Autodesk Inventor part; units mm, degrees
ref_plane "Plano de trabajo1" through (-18, 0, -54) normal (1, 0, 0) x (0, 0, -1)
ref_plane "YZ Plane" through (0, 0, 0) normal (1, 0, 0) x (0, 1, 0)
ref_plane "XZ Plane" through (0, 0, 0) normal (0, 1, 0) x (-1, 0, 0)
sketch "Boceto1" plane through (0, 0, 0) normal (0, 1, 0) x (-1, 0, 0)
  line L0 (-15, 60) -> (15, 60)
  line L1 (21, 54) -> (21, -54)
  line L2 (15, -60) -> (-15, -60)
  line L3 (-21, -54) -> (-21, 54)
  line L4 (-21, 60) -> (21, -60) construction
  line L5 (21, 60) -> (-21, -60) construction
  arc A0 (21, 54) -> (15, 60) centre (15, 54) ccw
  arc A1 (-15, 60) -> (-21, 54) centre (-15, 54) ccw
  arc A2 (-21, -54) -> (-15, -60) centre (-15, -54) ccw
  arc A3 (15, -60) -> (21, -54) centre (15, -54) ccw
  circle A4 centre (0, 46) radius 7.5
  circle A5 centre (0, -46) radius 7.5
  point P0 (0, 0)
  dimension "d0" = 42
  dimension "d1" = 120
  dimension "d2" = 6
  dimension "d3" = 15
  dimension "d13" = 46
  dimension "d14" = 46
extrude "Extrusión1" add sketch "Boceto1" along normal blind 10
sketch "Boceto2" plane through (-21, 0, -54) normal (-1, 0, 0) x (0, 0, 1)
  line L0 (0, 10) -> (108, 10) construction
  line L1 (24, 86.9722) -> (24, 26)
  line L2 (84, 86.9722) -> (84, 26)
  line L3 (0, 0) -> (108, 0)
  arc A0 (84, 26) -> (100, 10) centre (100, 26) ccw
  arc A1 (8, 10) -> (24, 26) centre (8, 26) ccw
  line L4 (92.5, 10) -> (107.5, 10) construction
  line L5 (0.5, 10) -> (15.5, 10) construction
  circle A2 centre (54, 105) radius 35
  line L6 (8, 10) -> (100, 10)
  point P0 (54, 0)
  point P1 (24, 10)
  point P2 (84, 10)
  point P3 (54, 0)
  point P4 (54, 0)
  point P5 (54, 10)
  dimension "d10" = 16
  dimension "d16" = 35
  dimension "d17" = 95
extrude "Extrusión2" add sketch "Boceto2" against normal blind 6 contours A2 L2 A0 L6 A1 L1
ref_plane "Plano de trabajo1" through (-18, 0, -54) normal (1, 0, 0) x (0, 0, -1)
sketch "Boceto3" plane through (-18, 0, -54) normal (1, 0, 0) x (0, 0, -1)
  arc A0 (-84, 86.9722) -> (-24, 86.9722) centre (-54, 105) ccw
  circle A1 centre (-54, 105) radius 35
  circle A2 centre (-54, 105) radius 30
  line L0 (-57, 10) -> (-51, 10)
  line L1 (-51, 10) -> (-51, 70.1288)
  line L2 (-51, 70.1288) -> (-57, 70.1288)
  line L3 (-57, 70.1288) -> (-57, 10)
  line L4 (-57, 10) -> (-51, 70.1288) construction
  line L5 (-51, 10) -> (-57, 70.1288) construction
  line L6 (-8, 10) -> (-100, 10)
  line L7 (-55.5, 105) -> (-52.5, 105)
  line L8 (-52.5, 105) -> (-52.5, 175)
  line L9 (-52.5, 175) -> (-55.5, 175)
  line L10 (-55.5, 175) -> (-55.5, 105)
  line L11 (-55.5, 105) -> (-52.5, 175) construction
  line L12 (-52.5, 105) -> (-55.5, 175) construction
  point P0 (-54, 0)
  point P1 (-54, 40.0644)
  point P2 (-54, 140)
  point P3 (-55.5, 134.9625)
  point P4 (-55.5, 139.9678)
  point P5 (-52.5, 139.9678)
  point P6 (-52.5, 134.9625)
  dimension "d23" = 39
  dimension "d20" = 30
  dimension "d21" = 6
  dimension "d22" = 3
extrude "Extrusión3" add sketch "Boceto3" along normal up to surface (39 mm away) contours A1 L10 A2 L8 A0 L2 | L2 A0 | A0 L1 L0 L3
sketch "Boceto4" plane through (-18, 0, -54) normal (-1, 0, 0) x (0, 0, 1)
  arc A0 (24, 86.9722) -> (84, 86.9722) centre (54, 105) ccw
  arc A1 (84, 86.9722) -> (55.5, 139.9678) centre (54, 105) ccw
  line L0 (55.5, 134.9625) -> (55.5, 139.9678)
  arc A2 (52.5, 134.9625) -> (55.5, 134.9625) centre (54, 105) ccw
  line L1 (52.5, 139.9678) -> (52.5, 134.9625)
  arc A3 (52.5, 139.9678) -> (24, 86.9722) centre (54, 105) ccw
  point P0 (54, 0)
extrude "Extrusión4" add sketch "Boceto4" along normal blind 9
sketch "Sketch6" plane through (-21, 0, -54) normal (-1, 0, 0) x (0, 0, 1)
  arc A0 (52.5, 139.9678) -> (55.5, 139.9678) centre (54, 105) ccw
  line L0 (52.5, 139.9678) -> (52.5, 161)
  line L1 (52.5, 161) -> (21.5, 161)
  line L2 (21.5, 161) -> (21.5, 117.9904)
  line L3 (21.5, 147) -> (52.5, 147) construction
  point P0 (54, 0)
  dimension "d30" = 31
  dimension "d31" = 42
  dimension "d32" = 14
extrude "Extrusion5" add sketch "Sketch6" against normal blind 28
fillet "Fillet1" radius 14 2 edges at (7, 161, -17) (-21, 161, -17)
sketch "Sketch7" plane through (7, 117.9904, -32.5) normal (0, 0, -1) x (-1, 0, 0)
  arc A0 (28, 29.0096) -> (0, 29.0096) centre (14, 29.0096) ccw
  point P0 (7, -117.9904)
hole "Hole1" at (-7, 147, -32.5) direction (0, 0, 1) diameter 12 depth 31
mirror "Mirror1" about plane through (0, 0, 0) normal (0, 0, 1) of "Extrusion5", "Fillet1", "Hole1"
sketch "Sketch8" plane through (0, 0, 0) normal (0, 0, 1) x (1, 0, 0)
  line L0 (-27, 70) -> (-21, 70)
  line L1 (-21, 0) -> (-21, 10)
  line L2 (-21, 10) -> (-21, 26)
  line L3 (-21, 26) -> (-21, 86.9722)
  line L4 (-21, 86.9722) -> (-21, 86.9722)
  line L5 (-21, 86.9722) -> (-21, 26)
  line L6 (-21, 26) -> (-21, 10)
  line L7 (-21, 0) -> (-21, 10)
  line L8 (-27, 70) -> (-21, 20)
  line L9 (-27, 139.9678) -> (-27, 70)
  line L10 (-27, 70) -> (-27, 73)
  line L11 (-27, 73) -> (-21, 73)
  point P0 (0, 0)
  dimension "d43" = 20
  dimension "d44" = 3
extrude "Extrusion6" add sketch "Sketch8" along normal mid plane 6
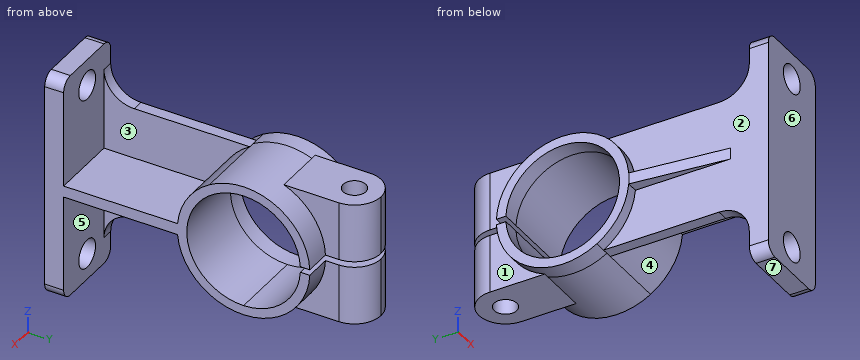
Input: part model. Units: mm. Frame: model coordinates. Face numbers are marked on the shaded views. A direction names the side the tool comes from. Coordinates: 2 decimals unless noted, no trailing zeros. Loops run counter-clockwise (first coordinate to the right, second up) from the corner with the lowest first, then second, coordinate; pieces in that order, holes last. Notation, with made-up numbers: (80.25, -36.75) -> (137.25, -36.75) arc R14 ccw to (137.25, -25.75) -> close; hole circle Ø10 at (75, 71.5). An arc over 180 degrees is marked (long way). Use a Markdown table: item, result.
1) Pull-direction query (Y, two-part tool) for the marked faces 5, 6 and 7; classes: released by +Y, released by -Y, zero draft, split by the parting line, or undercut.
Results found:
| item | result |
|---|---|
| face 5 | undercut |
| face 6 | released by -Y |
| face 7 | zero draft |
2) Cut plane D-D (y = 100.5). Return the cut outline in (x, z).
Results found:
| item | result |
|---|---|
| outline | (-27, -34.71) -> (21, -34.71) -> (21, -29.66) -> (-27, -29.66) -> close; (-27, 29.66) -> (21, 29.66) -> (21, 34.71) -> (-27, 34.71) -> close |
3) Access query for the marked faces 1, 2, 3 and 4. Directions: +Z, -Z, +X, -X, +Y, -Y. A direction counts if a zero-diameter tool reaches every point of the face in a straight line with its end or side. Return the directions, or none.
Results found:
| item | result |
|---|---|
| face 1 | -Z, -X, +Y |
| face 2 | -X, -Y |
| face 3 | +Z, +X |
| face 4 | -Z, +X |
4) Cut plane B-B (x = 2). Return the cut outline in (y, z).
Results found:
| item | result |
|---|---|
| outline | (0, -60) -> (10, -60) -> (10, -53.23) -> (0, -53.23) -> close; (0, -38.77) -> (10, -38.77) -> (10, -3) -> (70.13, -3) arc R35 ccw to (117.99, -32.5) -> (157.72, -32.5) -> (157.72, -1.5) -> (134.96, -1.5) arc R30 cw (long way) to (134.96, 1.5) -> (157.72, 1.5) -> (157.72, 32.5) -> (117.99, 32.5) arc R35 ccw to (86.97, 30) arc R35 ccw to (70.13, 3) -> (10, 3) -> (10, 38.77) -> (0, 38.77) -> close; (0, 53.23) -> (10, 53.23) -> (10, 60) -> (0, 60) -> close |
5) Contact query for flat-ended pins moving along their axis: pin 1 (1.5 mm diameter, centred on x = 10.5, z = 42, fed in from +Y); pin 2 (21 mm diameter, centred on x = -7.5, z = 38, fed in from +Y); pin 3 (19 mm diameter, centred on x = -7, y = 147, fed in from -Z); pin 4 (3 mm diameter, centred on x = -24.5, y = 56.5, fed in from +Z). Output: stop coordinate, or through.
Results found:
| item | result |
|---|---|
| pin 1 | stops at y = 10 |
| pin 2 | stops at y = 161 |
| pin 3 | stops at z = -32.5 |
| pin 4 | stops at z = 3 |
6) Cut plane C-C (y = 129.5). Return the cut outline in (x, z) (3 decimals), then the cut area to 3 significant figures.
Results found:
| item | result |
|---|---|
| outline | (-27, -24.995) -> (-21, -24.995) -> (-21, -32.5) -> (7, -32.5) -> (7, -24.995) -> (21, -24.995) -> (21, -17.313) -> (-27, -17.313) -> close; (-27, 17.313) -> (21, 17.313) -> (21, 24.995) -> (7, 24.995) -> (7, 32.5) -> (-21, 32.5) -> (-21, 24.995) -> (-27, 24.995) -> close |
| area | 1,160 mm2 |
7) Material intervals for line 1 along Z through (x, y) = (0, 6.5); line 2 along Z through (x, y) = (4, 154.5); line 3 along X through (y, z) = (147, -17), sorted ascending. Write a range as from..to.
Results found:
| item | result |
|---|---|
| line 1 | z = -60..-53.5, -38.5..38.5, 53.5..60 |
| line 2 | z = -32.5..-1.5, 1.5..32.5 |
| line 3 | x = -21..-13, -1..7 |
8) Cut plane A-A (z = 48). Return the cut outline in (x, y), then the cut area to 3 significant figures.
Results found:
| item | result |
|---|---|
| outline | (-21, 0) -> (-7.23, 0) -> (-7.23, 10) -> (-21, 10) -> close; (7.23, 0) -> (21, 0) -> (21, 10) -> (7.23, 10) -> close |
| area | 275 mm2 |
